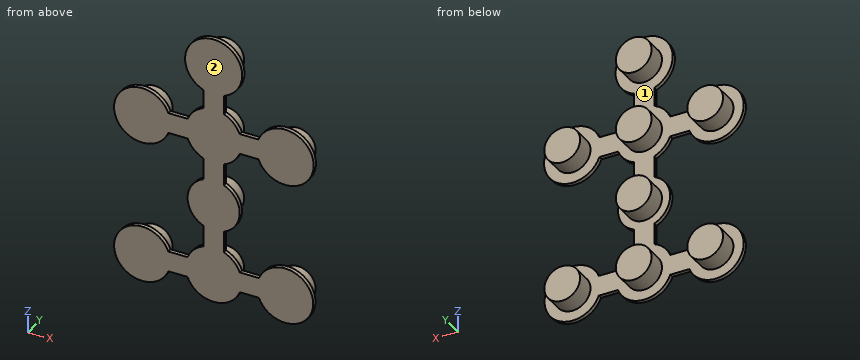
from build123d import *

# Parameters (mm, degrees)
BOSS_EXTRUDE1_DEPTH = 0.4
SKETCH2_R           = 1.75
BOSS_EXTRUDE2_DEPTH = 1.85


with BuildPart() as part:
    # Sketch1 → Boss-Extrude1 (new body)
    with BuildSketch(Plane(origin=(0, 0, 0), x_dir=(1, 0, 0), z_dir=(0, 1, 0))):
        with BuildLine():
            Line((2.561737691, 1), (4.438262309, 1))
            ThreePointArc((4.438262309, 1), (7, 2.75), (9.561737691, 1))
            Line((9.561737691, 1), (11.438262309, 1))
            ThreePointArc((11.438262309, 1), (16.75, 0), (11.438262309, -1))
            Line((11.438262309, -1), (9.561737691, -1))
            ThreePointArc((9.561737691, -1), (8.944543648, -1.944543648), (8, -2.561737691))
            Line((8, -2.561737691), (8, -4.647588392))
            ThreePointArc((8, -4.647588392), (9.556137785, -7), (8, -9.352411608))
            Line((8, -9.352411608), (8, -11.456717793))
            ThreePointArc((8, -11.456717793), (8.932392867, -12.067607133), (9.543282207, -13))
            Line((9.543282207, -13), (11.386254927, -13))
            ThreePointArc((11.386254927, -13), (16.798510909, -14), (11.386254927, -15))
            Line((11.386254927, -15), (9.543282207, -15))
            ThreePointArc((9.543282207, -15), (8.932392867, -15.932392867), (8, -16.543282207))
            Line((8, -16.543282207), (8, -18.386254927))
            ThreePointArc((8, -18.386254927), (7, -23.798510909), (6, -18.386254927))
            Line((6, -18.386254927), (6, -16.543282207))
            ThreePointArc((6, -16.543282207), (5.067607133, -15.932392867), (4.456717793, -15))
            Line((4.456717793, -15), (2.566233649, -15))
            ThreePointArc((2.566233649, -15), (-2.754188654, -14), (2.566233649, -13))
            Line((2.566233649, -13), (4.456717793, -13))
            ThreePointArc((4.456717793, -13), (5.067607133, -12.067607133), (6, -11.456717793))
            Line((6, -11.456717793), (6, -9.352411608))
            ThreePointArc((6, -9.352411608), (4.443862215, -7), (6, -4.647588392))
            Line((6, -4.647588392), (6, -2.561737691))
            ThreePointArc((6, -2.561737691), (5.055456352, -1.944543648), (4.438262309, -1))
            Line((4.438262309, -1), (2.561737691, -1))
            ThreePointArc((2.561737691, -1), (-2.75, 0), (2.561737691, 1))
        make_face()
    extrude(amount=BOSS_EXTRUDE1_DEPTH)

    # Sketch2 → Boss-Extrude2 (add)
    with BuildSketch(Plane(origin=(0, 0.4, 0), x_dir=(1, 0, 0), z_dir=(0, 1, 0))):
        with Locations(Location((0, 0, 0), (0, 0, 270))):
            Circle(SKETCH2_R)
        with Locations(Location((7, 0, 0), (0, 0, 270))):
            Circle(SKETCH2_R)
        with Locations(Location((14, 0, 0), (0, 0, 270))):
            Circle(SKETCH2_R)
        with Locations(Location((7, -7, 0), (0, 0, 270))):
            Circle(SKETCH2_R)
        with Locations(Location((7, -14, 0), (0, 0, 270))):
            Circle(SKETCH2_R)
        with Locations(Location((14, -14, 0), (0, 0, 270))):
            Circle(SKETCH2_R)
        with Locations(Location((0, -14, 0), (0, 0, 270))):
            Circle(SKETCH2_R)
        with Locations(Location((7, -21, 0), (0, 0, 270))):
            Circle(SKETCH2_R)
    extrude(amount=BOSS_EXTRUDE2_DEPTH)


solid = part.part
The listing builds one solid part. Answer for the finished solid, in the listing's coordinates (mm). Face numbers are marked on the shaded views. Coordinates: 2 decimals unless noted, no trailing zeros. Loops run counter-clockwise (first coordinate to the right, second up) from the corner with the lowest first, then second, coordinate; pieces in that order, holes last. Notation, with made-up numbers: (-27.5, -5) -> (3.5, -5) arc R23 ccw to (3.5, 33) -> close; hole circle Ø3 at (44, 87). An arc over 180 degrees is marked (long way). Answer in a Markdown table with one row per item. Add a question column.
1. The part is cut by section A-A, the plane x = 10.25. Write down the section's boundary in (y, z).
2. The part is cut by section C-C, the plane z = 0. Write down the section's boundary in (x, y).
3. Determine the mould class of the marked faces 1 and 2 for opening direction Z: +Z half, -Z half, draft (parallel to the pull), parting line (faces both ways), or undercut.
4. The part is cut by section D-D, the plane x = 14. Write down the section's boundary in (y, z).
5. The part is cut by section B-B, the plane y = 0.7. Write down the section's boundary in (x, z), then the cut area to 3 significant figures.
6. Flat-ended cylindrical pins translate along their axes: P1, Ø10, axis at x = 11, z = 6, coming from the +Y side; P2, Ø1.5, axis at x = 9.5, z = 16.5, coming from the +Y side. Find the tip coordinate at first contact, or state that the pin passes through.
7. Consider line 1 (X direction, y = 0.8, z = 1.25); line 2 (Z direction, x = 5.5, y = 1.6); line 3 (Z direction, x = 7.5, y = 1.4). Determine where each line is inside the solid, lowest interval first. Write a range as [from, to].
Answer below:
| question | item | result |
|---|---|---|
| 1 | outline | (0, -1) -> (0.4, -1) -> (0.4, 1) -> (0, 1) -> close; (0, 13) -> (0.4, 13) -> (0.4, 15) -> (0, 15) -> close |
| 2 | outline | (-2.75, 0) -> (16.75, 0) -> (16.75, 0.4) -> (15.75, 0.4) -> (15.75, 2.25) -> (12.25, 2.25) -> (12.25, 0.4) -> (8.75, 0.4) -> (8.75, 2.25) -> (5.25, 2.25) -> (5.25, 0.4) -> (1.75, 0.4) -> (1.75, 2.25) -> (-1.75, 2.25) -> (-1.75, 0.4) -> (-2.75, 0.4) -> close |
| 3 | face 1 | undercut |
| 3 | face 2 | draft |
| 4 | outline | (0, -2.75) -> (0.4, -2.75) -> (0.4, -1.75) -> (2.25, -1.75) -> (2.25, 1.75) -> (0.4, 1.75) -> (0.4, 2.75) -> (0, 2.75) -> close; (0, 11.2) -> (0.4, 11.2) -> (0.4, 12.25) -> (2.25, 12.25) -> (2.25, 15.75) -> (0.4, 15.75) -> (0.4, 16.8) -> (0, 16.8) -> close |
| 5 | outline | circle Ø3.5 at (0, 0); circle Ø3.5 at (0, 14); circle Ø3.5 at (7, 0); circle Ø3.5 at (7, 7); circle Ø3.5 at (7, 14); circle Ø3.5 at (7, 21); circle Ø3.5 at (14, 0); circle Ø3.5 at (14, 14) |
| 5 | area | 77.0 mm2 |
| 6 | P1 | y = 2.25 |
| 6 | P2 | through |
| 7 | line 1 | [-1.22, 1.22], [5.78, 8.22], [12.78, 15.22] |
| 7 | line 2 | [-0.9, 0.9], [6.1, 7.9], [13.1, 14.9], [20.1, 21.9] |
| 7 | line 3 | [-1.68, 1.68], [5.32, 8.68], [12.32, 15.68], [19.32, 22.68] |
